```python
from build123d import *

# Parameters (mm, degrees)
SKETCH_1_W          = 40
SKETCH_1_H          = 20
EXTRUDE_1_DEPTH     = 10
SKETCH_2_R          = 3.07375
CUT_EXTRUDE_1_DEPTH = 10
EXTRUDE_2_DEPTH     = 40
CUT_EXTRUDE_2_DEPTH = 92.624619881
SKETCH_5_W          = 5
SKETCH_5_H          = 17
CUT_EXTRUDE_3_DEPTH = 91.450654881
CHAMFER_1_SIZE      = 5
CHAMFER_2_SIZE      = 2


with BuildPart() as part:
    # 草图1 → 凸台-拉伸1 (new body)
    with BuildSketch(Plane(origin=(0, 0, 0), x_dir=(0, 0, -1), z_dir=(1, 0, 0))):
        with Locations((20, 10)):
            Rectangle(SKETCH_1_W, SKETCH_1_H)
    extrude(amount=EXTRUDE_1_DEPTH)

    # 草图2 → 切除-拉伸1 (cut)
    with BuildSketch(Plane(origin=(10, 0, 0), x_dir=(0, 0, -1), z_dir=(1, 0, 0))):
        with Locations((11.75, 10)):
            Circle(SKETCH_2_R)
        with Locations((29.25, 10)):
            Circle(SKETCH_2_R)
    extrude(amount=-CUT_EXTRUDE_1_DEPTH, mode=Mode.SUBTRACT)

    # 草图3 → 凸台-拉伸2 (add)
    with BuildSketch(Plane(origin=(0, 0, -40), x_dir=(-1, 0, 0), z_dir=(0, 0, -1))):
        Polygon((0, 20), (0, 46.899019914), (13.875, 46.899019914), (13.875, 78.899019914), (8.875, 78.899019914), (8.875, 51.899019914), (-10, 51.899019914), (-10, 20), align=None)
    extrude(amount=-EXTRUDE_2_DEPTH)

    # 草图4 → 切除-拉伸2 (cut, through all)
    with BuildSketch(Plane(origin=(10, 0, 0), x_dir=(0, 0, -1), z_dir=(1, 0, 0))):
        Polygon((30, 30), (30, 88.448191602), (51.195528036, 88.448191602), (51.195528036, 8.804471964), align=None)
        Polygon((10, 30), (10, 90.801384447), (0, 90.801384447), (0, 20), align=None)
    extrude(amount=-CUT_EXTRUDE_2_DEPTH, mode=Mode.SUBTRACT)

    # 草图5 → 切除-拉伸3 (cut, through all)
    with BuildSketch(Plane(origin=(-8.875, 0, 0), x_dir=(0, 0, -1), z_dir=(1, 0, 0))):
        with Locations((12.5, 70.399019914)):
            Rectangle(SKETCH_5_W, SKETCH_5_H)
        with Locations((27.5, 70.399019914)):
            Rectangle(SKETCH_5_W, SKETCH_5_H)
    extrude(amount=-CUT_EXTRUDE_3_DEPTH, mode=Mode.SUBTRACT)

    # 倒角1
    chamfer_1_edges = [part.edges().sort_by_distance(p)[0] for p in [
        (-11.375, 61.899019914, -25),
        (-11.375, 61.899019914, -15),
    ]]
    chamfer(chamfer_1_edges, length=CHAMFER_1_SIZE - 0.0001)  # a hair under: the kernel refuses the full size

    # 倒角2
    chamfer_2_edges = [part.edges().sort_by_distance(p)[0] for p in [
        (-11.375, 78.899019914, -15),
        (-11.375, 78.899019914, -25),
    ]]
    chamfer(chamfer_2_edges, length=CHAMFER_2_SIZE)


solid = part.part
```
Geometry check sheet. Reference: the model listing, model coordinates, mm. A direction names the side the tool comes from. Give positions to 0.01 mm unless a question says otherwise; leave off trailing zeros. Order: outer loops, then holes, each group sorted by start corner. A loop starts at its lowest first (then second) coordinate and runs counter-clockwise, first axis right, second up. Notation, with made-up numbers: (-22, 72.5) - (12, 72.5) arc R15 ccw to (12, 93.5) - close; hole circle Ø9 at (-12.75, 38). An arc over 180 degrees is marked (long way). Answer in a Markdown table with one row per item. Add a question column.
Q1. Cross-section at C-C, the plane z = -29.25. Enter the section's corners in (x, y) (3 decimals), then the cut area to 3 significant figures.
Q2. Material ranges on probe 1 along Y at (x, z) = (5.75, -12); probe 2 along X at (y, z) = (38, -21.5); probe 3 along X at (y, z) = (65, -25.5) (3 decimals), recorded low to high. Write a range as from..to.
Q3. Cross-section at A-A, the plane y = 10. Enter the section's corners in (x, z), then the cut area to 3 significant figures.
Q4. Cross-section at B-B, the plane x = 3.5. Enter the section's corners in (y, z), then the cut area to 3 significant figures.
Q5. Mould release check, pull along Z, two halves, no side actions. Record for faces 1 (the cylindrical face through (5.07, 8.82, -32.09)), 2 (the flat face through (5, 0, -20)), 3 (the flat face through (5, 25, -35)): pulls with the +Z half, pulls with the -Z half, needs draft (parallel to the pull), parting line crosses it, or undercut.
Q6. Tool access check on faces 4 (the flat face through (1, 46, -10)), 5 (the flat face through (1, 46, -30)), 6 (the flat face through (0, 51.899, -20)), 7 (the flat face through (-7, 46.899, -20)), 8 (the flat face through (-13.875, 59, -20)). Record the directions out of +Z, -Z, +X, -X, +Y, -Y that give a thin tool (end or side, any length) a straight path to the whole face; none if there is none.
Q7. Cross-section at D-D, the plane z = -5. Enter the section's corners in (x, y).
Q8. Gauge pin test, flat ends, axial feed: pin 1 (3.5 mm diameter, centred on y = 10, z = -29.25, fed in from +X); pin 2 (7 mm diameter, centred on x = 0, y = 40, fed in from -Z); pin 3 (11 mm diameter, centred on x = -8, z = -18.5, fed in from -Y); pin 4 (12 mm diameter, centred on x = 3, y = 42, fed in from +Z). Record the tip position at first contact, or that the pin passes through.
Check values:
| question | item | result |
|---|---|---|
| 1 | outline | (-13.875, 46.899) - (0, 46.899) - (0, 13.074) - (10, 13.074) - (10, 51.899) - (-8.875, 51.899) - (-8.875, 62.649) - (-13.875, 62.649) - close; (0, 0) - (10, 0) - (10, 6.926) - (0, 6.926) - close |
| 1 | area | 581 mm^2 |
| 2 | probe 1 | y = 0..6.94, 13.06..51.9 |
| 2 | probe 2 | x = 0..10 |
| 2 | probe 3 | x = -13.875..-8.875 |
| 3 | outline | (0, -40) - (10, -40) - (10, -32.32) - (0, -32.32) - close; (0, -26.18) - (10, -26.18) - (10, -14.82) - (0, -14.82) - close; (0, -8.68) - (10, -8.68) - (10, 0) - (0, 0) - close |
| 3 | area | 277 mm^2 |
| 4 | outline | (0, -40) - (20, -40) - (30, -30) - (51.9, -30) - (51.9, -10) - (30, -10) - (20, 0) - (0, 0) - close; hole circle Ø6.15 at (10, -29.25); hole circle Ø6.15 at (10, -11.75) |
| 4 | area | 1,480 mm^2 |
| 5 | face 1 | undercut |
| 5 | face 2 | needs draft |
| 5 | face 3 | pulls with the -Z half |
| 6 | face 4 | +Z, +X, -X, +Y |
| 6 | face 5 | -Z, +X, -X, +Y |
| 6 | face 6 | +Z, -Z, +X, +Y |
| 6 | face 7 | +Z, -Z, -X, -Y |
| 6 | face 8 | +Z, -Z, -X, +Y, -Y |
| 7 | outline | (0, 0) - (10, 0) - (10, 25) - (0, 25) - close |
| 8 | pin 1 | passes through |
| 8 | pin 2 | stops at z = -30 |
| 8 | pin 3 | stops at y = 46.9 |
| 8 | pin 4 | stops at z = -10 |
